Geometry: final body of the model. Coordinates: model frame, mm. Round coordinates to 2 decimals unless told otherwise and drop trailing zeros. Loops run counter-clockwise (first coordinate to the right, second up) from the corner with the lowest first, then second, coordinate; pieces in that order, holes last. Notation, with made-up numbers: (-13, 66.25) - (26, 66.25) arc R7 ccw to (26, 74.25) - close; hole circle Ø5 at (52.5, 54). An arc over 180 degrees is marked (long way). Write item = value, one per line. Start each with the question number.
Item 1: Section C-C (z = 3.1). Count the separate pieces of the cut face and the enclosed holes in it, plus the area to 3 significant figures.
Item 2: Section B-B (y = 0). Return loops of the section in (x, z) (3 decimals), plus the area to 3 significant figures.
Item 3: First-contact query: pin 1 (10 mm diameter, centred on x = 3, y = 28.5, fed in from +Z); pin 2 (1 mm diameter, centred on x = 8, z = 2.5, fed in from +Y); pin 3 (1 mm diameter, centred on x = 36.5, z = 3.5, fed in from +Y). Flat tips, straight axial feed; report the tip coordinate or a pass-through.
Item 4: Line query: line 1 (Y direction, x = 23.5, z = 2.3); line 2 (Y direction, x = 0, z = 1.2); line 3 (Y direction, x = 23.5, z = 1.3). Output: solid intervals per line, ascending. Write a range as from..to.
Item 5: Section D-D (x = -23.5). Return loops of the section in (y, z), plus the area to 3 significant figures.
Item 6: Section A-A (x = 0). Return loops of the section in (y, z), plus the area to 3 significant figures.
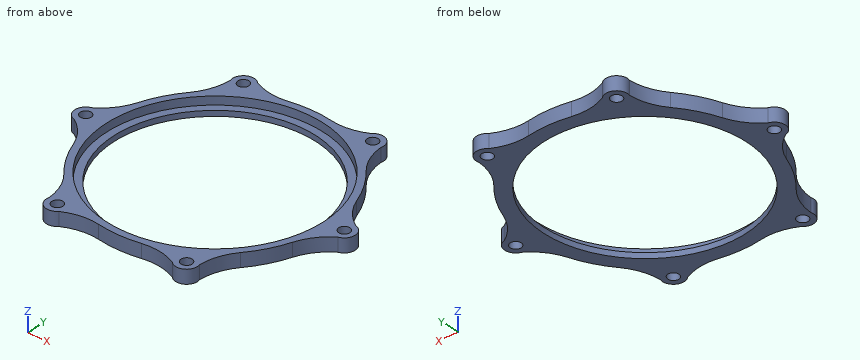
from build123d import *

# Parameters (mm, degrees)
F0_R     = 39.75
F0_R_2   = 37
F1_DEPTH = 2
F0_R_3   = 2.025
F2_DEPTH = 5


with BuildPart() as f1:
    # F0 (on Top) → F1 (new body)
    with BuildSketch(Plane.XY):
        Circle(F0_R)
        Circle(F0_R_2, mode=Mode.SUBTRACT)
    extrude(amount=F1_DEPTH)

    # F0 (on Top) → F2 (join)
    with BuildSketch(Plane.XY):
        with BuildLine():
            ThreePointArc((-27.354102, 39.632728), (-28.694314, 33.185179), (-32.055879, 27.522411))
            ThreePointArc((-32.055879, 27.522411), (-36.589573, 21.125), (-39.863047, 14))
            ThreePointArc((-39.863047, 14), (-43.086364, 8.257415), (-48, 3.872983))
            ThreePointArc((-48, 3.872983), (-51, 0), (-48, -3.872983))
            ThreePointArc((-48, -3.872983), (-43.086364, -8.257415), (-39.863047, -14))
            ThreePointArc((-39.863047, -14), (-36.589573, -21.125), (-32.055879, -27.522411))
            ThreePointArc((-32.055879, -27.522411), (-28.694314, -33.185179), (-27.354102, -39.632728))
            ThreePointArc((-27.354102, -39.632728), (-25.5, -44.167296), (-20.645898, -43.505711))
            ThreePointArc((-20.645898, -43.505711), (-14.392051, -41.442594), (-7.807168, -41.522411))
            ThreePointArc((-7.807168, -41.522411), (0, -42.25), (7.807168, -41.522411))
            ThreePointArc((7.807168, -41.522411), (14.392051, -41.442594), (20.645898, -43.505711))
            ThreePointArc((20.645898, -43.505711), (25.5, -44.167296), (27.354102, -39.632728))
            ThreePointArc((27.354102, -39.632728), (28.694314, -33.185179), (32.055879, -27.522411))
            ThreePointArc((32.055879, -27.522411), (36.589573, -21.125), (39.863047, -14))
            ThreePointArc((39.863047, -14), (43.086364, -8.257415), (48, -3.872983))
            ThreePointArc((48, -3.872983), (51, 0), (48, 3.872983))
            ThreePointArc((48, 3.872983), (43.086364, 8.257415), (39.863047, 14))
            ThreePointArc((39.863047, 14), (36.589573, 21.125), (32.055879, 27.522411))
            ThreePointArc((32.055879, 27.522411), (28.694314, 33.185179), (27.354102, 39.632728))
            ThreePointArc((27.354102, 39.632728), (25.5, 44.167296), (20.645898, 43.505711))
            ThreePointArc((20.645898, 43.505711), (14.392051, 41.442594), (7.807168, 41.522411))
            ThreePointArc((7.807168, 41.522411), (0, 42.25), (-7.807168, 41.522411))
            ThreePointArc((-7.807168, 41.522411), (-14.392051, 41.442594), (-20.645898, 43.505711))
            ThreePointArc((-20.645898, 43.505711), (-25.5, 44.167296), (-27.354102, 39.632728))
        make_face()
        with Locations((-23.5, -40.703194)):
            Circle(F0_R_3, mode=Mode.SUBTRACT)
        with Locations((23.5, -40.703194)):
            Circle(F0_R_3, mode=Mode.SUBTRACT)
        with Locations((-47, 0)):
            Circle(F0_R_3, mode=Mode.SUBTRACT)
        with Locations((-23.5, 40.703194)):
            Circle(F0_R_3, mode=Mode.SUBTRACT)
        Circle(F0_R, mode=Mode.SUBTRACT)
        with Locations((47, 0)):
            Circle(F0_R_3, mode=Mode.SUBTRACT)
        with Locations((23.5, 40.703194)):
            Circle(F0_R_3, mode=Mode.SUBTRACT)
    extrude(amount=F2_DEPTH)


solid = f1.part
Taken from the geometry:
q1.separate_pieces = 1
q1.enclosed_holes = 7
q1.area = 1,160 mm^2
q2.outline = (-51, 0) - (-49.025, 0) - (-49.025, 5) - (-51, 5) - close; (-44.975, 0) - (-37, 0) - (-37, 2) - (-39.75, 2) - (-39.75, 5) - (-44.975, 5) - close; (37, 0) - (44.975, 0) - (44.975, 5) - (39.75, 5) - (39.75, 2) - (37, 2) - close; (49.025, 0) - (51, 0) - (51, 5) - (49.025, 5) - close
q2.area = 83.0 mm^2
q3.pin_1 = through
q3.pin_2 = 41.58
q3.pin_3 = 22.11
q4.line_1 = -44.7..-42.73, -38.68..-32.06, 32.06..38.68, 42.73..44.7
q4.line_2 = -42.25..-37, 37..42.25
q4.line_3 = -44.7..-42.73, -38.68..-28.58, 28.58..38.68, 42.73..44.7
q5.outline = (-44.7, 0) - (-42.73, 0) - (-42.73, 5) - (-44.7, 5) - close; (-38.68, 0) - (-28.58, 0) - (-28.58, 2) - (-32.06, 2) - (-32.06, 5) - (-38.68, 5) - close; (28.58, 0) - (38.68, 0) - (38.68, 5) - (32.06, 5) - (32.06, 2) - (28.58, 2) - close; (42.73, 0) - (44.7, 0) - (44.7, 5) - (42.73, 5) - close
q5.area = 99.9 mm^2
q6.outline = (-42.25, 0) - (-37, 0) - (-37, 2) - (-39.75, 2) - (-39.75, 5) - (-42.25, 5) - close; (37, 0) - (42.25, 0) - (42.25, 5) - (39.75, 5) - (39.75, 2) - (37, 2) - close
q6.area = 36.0 mm^2
